Answer from the drawing. Dimensions are ordinates in mm from the lowest x, y and z of the part. A direction names the side the tool comes from. Round coordinates to 2 decimals unless told otherwise and drop trailing zeros. Loops run counter-clockwise (first coordinate to the right, second up) from the corner with the lowest first, then second, coordinate; pieces in that order, holes last.
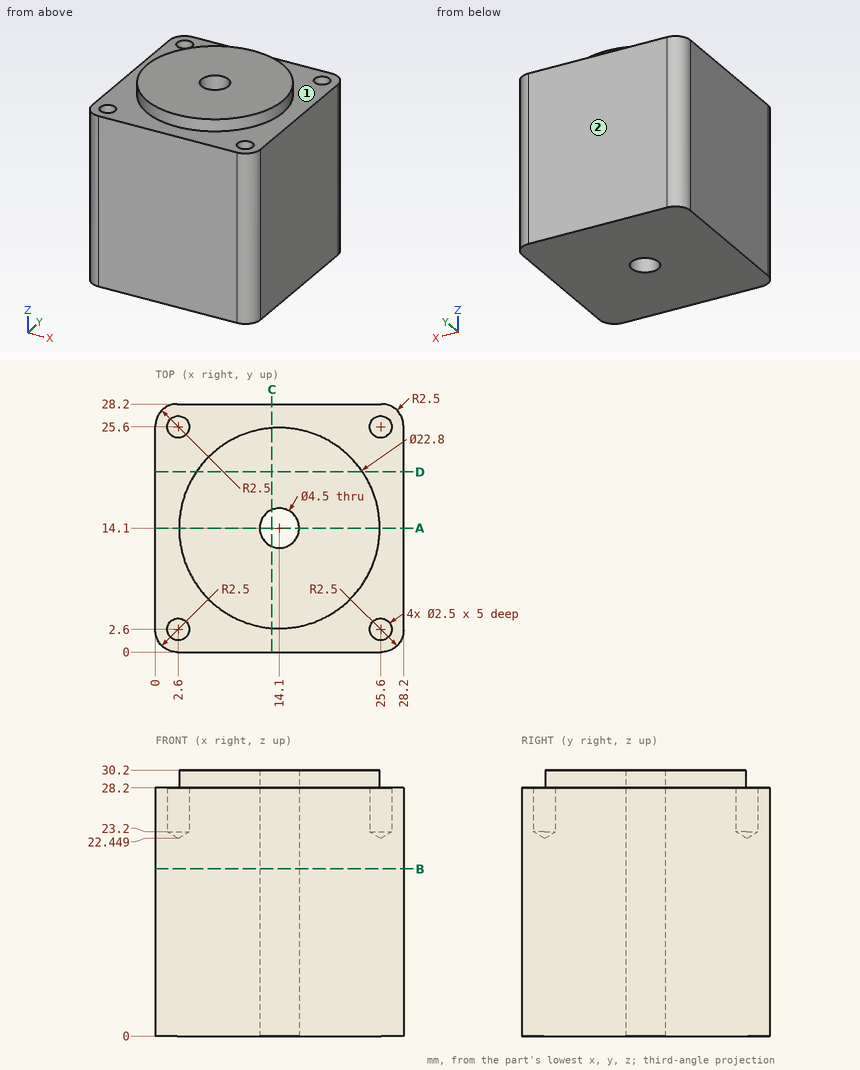
1. Which of the six approach directions +Z, -Z, +X, -X, +Y, -Y give full straight-line access (tool end or side, diameter ignored) to the marked faces 1 and 2?
Answer key:
face 1: +Z
face 2: +Z, -Z, +X, -X, +Y
2. Find section C-C (x = 13.25). Write down the section's boundary in (y, z).
Answer key:
outline: (0, 0) - (12.02, 0) - (12.02, 30.2) - (2.73, 30.2) - (2.73, 28.2) - (0, 28.2) - close; (16.18, 0) - (28.2, 0) - (28.2, 28.2) - (25.47, 28.2) - (25.47, 30.2) - (16.18, 30.2) - close
3. Find section D-D (y = 20.5). Write down the section's boundary in (x, z).
Answer key:
outline: (0, 0) - (28.2, 0) - (28.2, 28.2) - (23.53, 28.2) - (23.53, 30.2) - (4.67, 30.2) - (4.67, 28.2) - (0, 28.2) - close
4. Find section A-A (y = 14.1). Write down the section's boundary in (x, z), then the cut area to 3 significant figures.
Answer key:
outline: (0, 0) - (11.85, 0) - (11.85, 30.2) - (2.7, 30.2) - (2.7, 28.2) - (0, 28.2) - close; (16.35, 0) - (28.2, 0) - (28.2, 28.2) - (25.5, 28.2) - (25.5, 30.2) - (16.35, 30.2) - close
area: 705 mm2
5. Consider probe 1 along X at (y, z) = (2.6, 26.8); probe 2 along X at (y, z) = (14, 19.5). Determine where each line is inside the solid, lowest interval first.
Answer key:
probe 1: x = 0 to 1.35, 3.85 to 24.35, 26.85 to 28.2
probe 2: x = 0 to 11.85, 16.35 to 28.2
6. Given pin 1 (3 mm diameter, centred on x = 25.6, y = 2.6, fed in from +Z), flat-ended and moving along its own axis, determine where the tip first touches the part or whether it passes through.
Answer key:
pin 1: stops at z = 28.2
7. Find section B-B (z = 19). Write down the section's boundary in (x, y).
Answer key:
outline: (0, 2.5) arc R2.5 ccw to (2.5, 0) - (25.7, 0) arc R2.5 ccw to (28.2, 2.5) - (28.2, 25.7) arc R2.5 ccw to (25.7, 28.2) - (2.5, 28.2) arc R2.5 ccw to (0, 25.7) - close; hole circle Ø4.5 at (14.1, 14.1)
